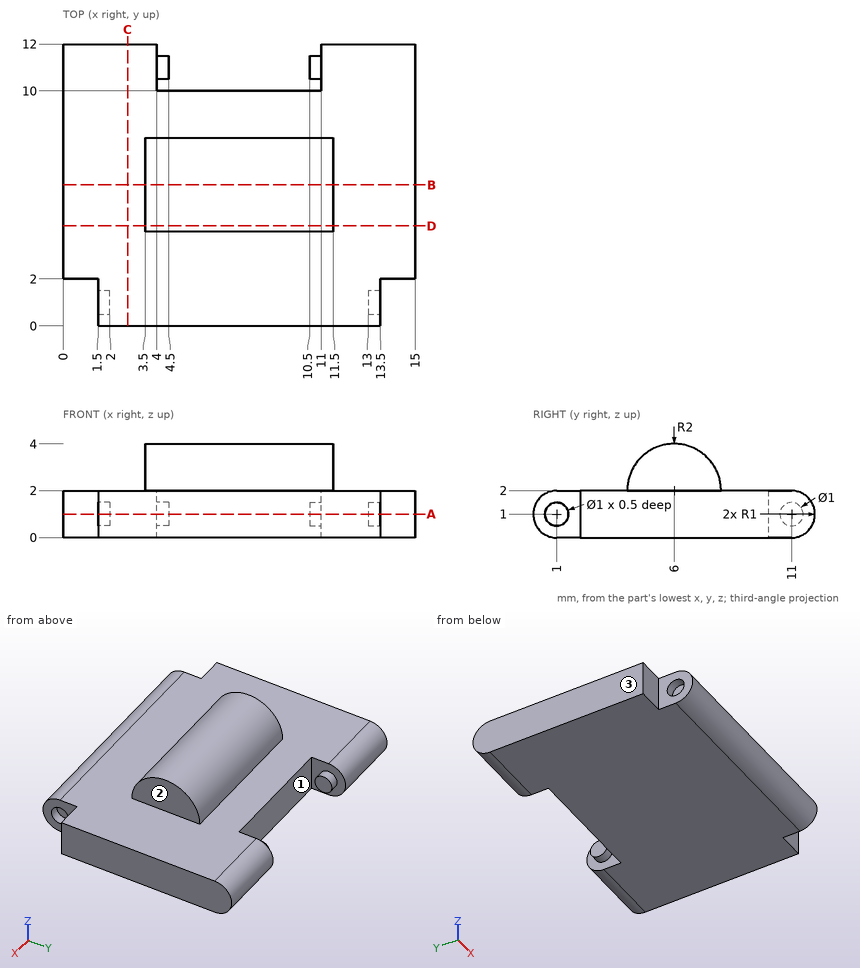
Study the drawing (mm; zero at the part's minimum x, y, z) and answer. Give positions to 0.01 mm unless a question says otherwise; leave off trailing zeros. Order: outer loops, then holes, each group sorted by start corner. A loop starts at its lowest first (then second) coordinate and runs counter-clockwise, first axis right, second up.
1) Find section B-B on y = 6. Write down the section's boundary in (x, z), then the cut area to 3 significant figures.
Reported:
outline: (0, 0) - (15, 0) - (15, 2) - (11.5, 2) - (11.5, 4) - (3.5, 4) - (3.5, 2) - (0, 2) - close
area: 46.0 mm2
2) Find section A-A on z = 1. Write down the section's boundary in (x, y).
Reported:
outline: (0, 2) - (1.5, 2) - (1.5, 1.5) - (2, 1.5) - (2, 0.5) - (1.5, 0.5) - (1.5, 0) - (13.5, 0) - (13.5, 0.5) - (13, 0.5) - (13, 1.5) - (13.5, 1.5) - (13.5, 2) - (15, 2) - (15, 12) - (11, 12) - (11, 11.5) - (10.5, 11.5) - (10.5, 10.5) - (11, 10.5) - (11, 10) - (4, 10) - (4, 10.5) - (4.5, 10.5) - (4.5, 11.5) - (4, 11.5) - (4, 12) - (0, 12) - close
3) Given P1, Ø0.8, axis at x = 14.5, z = 1, coming from the -Y side; P2, Ø1.5, axis at y = 3, z = 3, coming from the -X side; P3, Ø1.1, axis at y = 1, z = 1, coming from the -X side; P4, Ø1, axis at y = 6, z = 3, coming from the +X side, each flat-ended and moving along its own axis, determine where each tip first touches the part or whether it passes through.
Reported:
P1: stops at y = 2
P2: passes through
P3: stops at x = 1.5
P4: stops at x = 11.5
4) Determine the mould class of the marked faces 1, 2 and 3 for opening direction X: pulls with the +X half, pulls with the -X half, needs draft (parallel to the pull), parting line crosses it, or undercut.
Reported:
face 1: undercut
face 2: pulls with the +X half
face 3: pulls with the -X half
5) Find section C-C on x = 2.75. Write down the section's boundary in (y, z), then the cut area to 3 significant figures.
Reported:
outline: (1, 0) - (11, 0) arc R1 ccw to (11, 2) - (1, 2) arc R1 ccw to start
area: 23.1 mm2
6) Find section D-D on y = 4.25. Write down the section's boundary in (x, z).
Reported:
outline: (0, 0) - (15, 0) - (15, 2) - (11.5, 2) - (11.5, 2.97) - (3.5, 2.97) - (3.5, 2) - (0, 2) - close
7) Consider line 1 along X through (y, z) = (11, 1.4); line 2 along X through (y, z) = (4.5, 2.95); line 3 along Z through (x, y) = (6.75, 9.25). Determine where each line is inside the solid, lowest interval first.
Reported:
line 1: x = 0 to 4.5, 10.5 to 15
line 2: x = 3.5 to 11.5
line 3: z = 0 to 2
